Design review of the part built by this model. Coordinates are the model's own, in mm. A direction names the side the tool comes from. Coordinates: 2 decimals unless noted, no trailing zeros. Loops run counter-clockwise (first coordinate to the right, second up) from the corner with the lowest first, then second, coordinate; pieces in that order, holes last. Notation, with made-up numbers: M 84,36.5 L 114,36.5 A28 ccw 114,71.5 Z; hole C -10,8 d10. An arc over 180 degrees is marked long. Answer as a JSON object with one key per item and string values. Group by question number.
1. To check wall thickness, follow probe 1 along X at (y, z) = (-0.3, 1.8); probe 2 along Y at (x, z) = (-27, -0.05); probe 3 along Y at (x, z) = (-26.5, 0.45). State the ranges of each line that lie inside material, in increasing order.
2. Consider section C-C (x = -16). State the section outline as (y, z) points.
3. Machinability: for faces 1 (the cylindrical face through (-9.8, -0.45, 1.43)), 2 (the cylindrical face through (-13.75, -0.06, -1.45)), 3 (the cylindrical face through (-17, 2, 0)), which of the approach directions +Z, -Z, +X, -X, +Y, -Y give a long, thin tool a straight path to every point of the face, cutting with its end or side? Answer none if there is none.
4. Consider section A-A (z = 0). State the section outline as (x, y) points (3 decimals), then the cut area to 3 significant figures.
5. Draft analysis for pull direction X (two halves, no side actions). For faces 4 (the flat face through (0, 0, 0)), 5 (the cylindrical face through (-29.78, -0.45, 1.43)), 6 (the flat face through (-39, 0, 0)), 7 (the cylindrical face through (-20.25, -0.06, -1.45)), state which applies: +X half, -X half, draft (parallel to the pull), parting line (faces both ways), or undercut.
6. Insertion check: pin 1 (2 mm diameter, centred on x = -5.5, y = 0, fed in from -Z). The pin has a flat end and moves straight along its axis. Give the tip position at first contact, or say it passes through.
7. Consider section D-D (x = -23). State the section outline as (y, z) points.
from build123d import *

# Parameters (mm, degrees)
CHAMFER_1_SIZE = 0.2


with BuildPart() as part:
    # 草图1 → 旋转1 (revolve)
    with BuildSketch(Plane.XY, mode=Mode.PRIVATE) as revolve_1_sk:
        Polygon((0, 0), (0, 1.475), (-6, 1.475), (-6, 1.5), (-13.5, 1.5), (-13.5, 1.45), (-14, 1.45), (-14, 2), (-20, 2), (-20, 1.45), (-20.5, 1.45), (-20.5, 1.5), (-39, 1.5), (-39, 0), align=None)
    revolve(revolve_1_sk.sketch.rotate(Axis((-12.088767593, 0, 0), (1, 0, 0)), 90), axis=Axis((-12.088767593, 0, 0), (1, 0, 0)))

    # 倒角1
    chamfer_1_edges = [part.edges().sort_by_distance(p)[0] for p in [
        (0, 0, -1.475),
        (-39, 0, -1.5),
    ]]
    chamfer(chamfer_1_edges, length=CHAMFER_1_SIZE)


solid = part.part
Findings below:
{
 "1": {"probe 1": "x = -20 to -14", "probe 2": "y = -1.5 to 1.5", "probe 3": "y = -1.43 to 1.43"},
 "2": {"outline": "C 0,0 d4"},
 "3": {"face 1": "+X", "face 2": "none", "face 3": "+X, -X"},
 "4": {"outline": "M -39,-1.3 L -38.8,-1.5 L -20.5,-1.5 L -20.5,-1.45 L -20,-1.45 L -20,-2 L -14,-2 L -14,-1.45 L -13.5,-1.45 L -13.5,-1.5 L -6,-1.5 L -6,-1.475 L -0.2,-1.475 L 0,-1.275 L 0,1.275 L -0.2,1.475 L -6,1.475 L -6,1.5 L -13.5,1.5 L -13.5,1.45 L -14,1.45 L -14,2 L -20,2 L -20,1.45 L -20.5,1.45 L -20.5,1.5 L -38.8,1.5 L -39,1.3 Z", "area": "123 mm^2"},
 "5": {"face 4": "+X half", "face 5": "draft", "face 6": "-X half", "face 7": "undercut"},
 "6": {"pin 1": "stops at z = -1.5"},
 "7": {"outline": "C 0,0 d3"}
}
